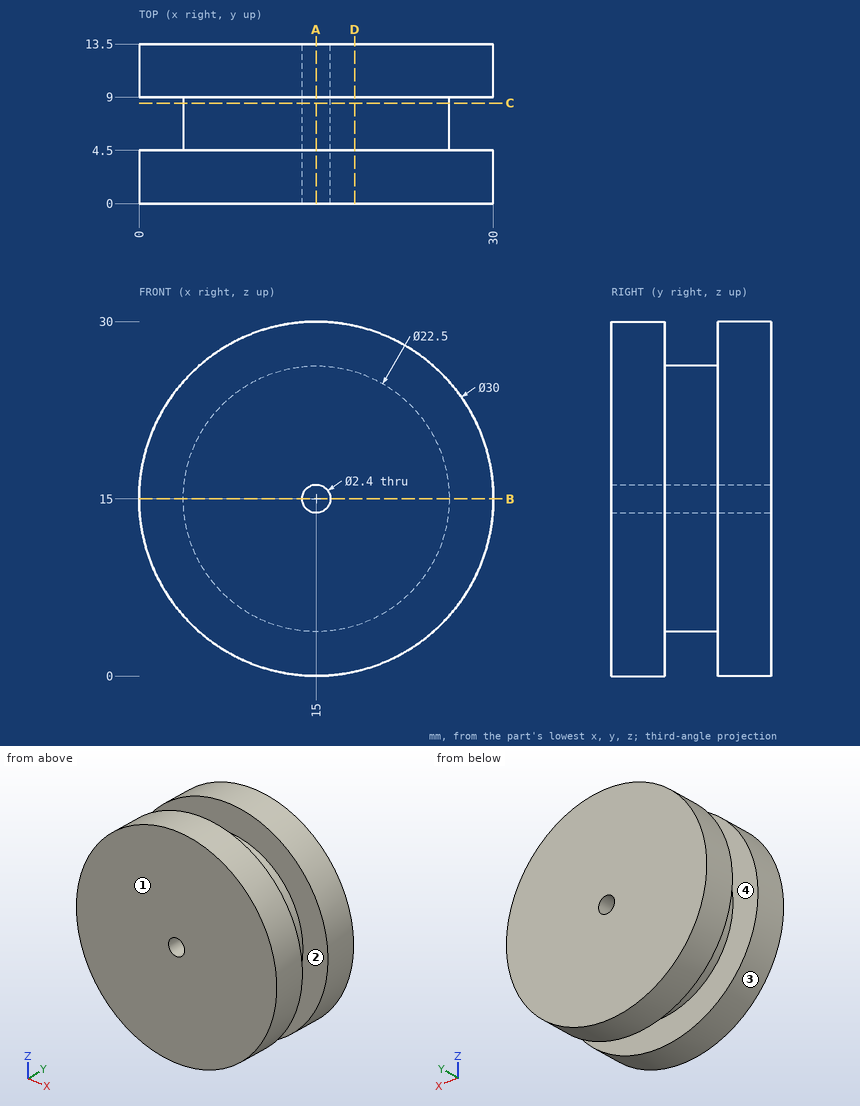
Geometry: see drawing. Coordinates: mm, zero at the bounding-box minimum. Coordinates: 2 decimals unless noted, no trailing zeros. Order: outer loops, then holes, each group sorted by start corner. A loop starts at its lowest first (then second) coordinate and runs counter-clockwise, first axis right, second up. Notation, with made-up numbers: M 82,83 L 98,83 A36 cw 98,121 Z; hole C 8,65.25 d5. An arc over 180 degrees is marked long. Write item = value, one per line. Start each with the question number.
(1) Pull-direction query (Y, two-part tool) for the marked faces 1, 2, 3 and 4; classes: released by +Y, released by -Y, zero draft, split by the parting line, or undercut.
(2) Section C-C on y = 8.5. Output: boundary loops of the cut face in (x, z), and give its area (3 significant figures).
(3) Line query: line 1 along X through (y, z) = (5.25, 15); line 2 along Y through (x, z) = (27.5, 20.5); line 3 along Z through (x, y) = (15, 9.5). Output: solid intervals per line, ascending. Write a range as [from, to].
(4) Section A-A on x = 15. Output: boundary loops of the cut face in (y, z).
(5) Section B-B on z = 15. Output: boundary loops of the cut face in (x, y).
(6) Section D-D on x = 18.25. Output: boundary loops of the cut face in (y, z).
(7) First-contact query: P1, Ø3, axis at x = 15, z = 15, coming from the -Y side; P2, Ø2, axis at x = 18.5, y = 11, coming from the -Z side; P3, Ø2, axis at x = 26, y = 12, coming from the +Z side; P4, Ø3, axis at x = 8, y = 9, coming from the -Z side. Flat tips, straight axial feed; report the tip coordinate or a pass-through.
Result set:
q1.face_1 = released by -Y
q1.face_2 = undercut
q1.face_3 = zero draft
q1.face_4 = undercut
q2.outline = C 15,15 d22.5; hole C 15,15 d2.4
q2.area = 393 mm²
q3.line_1 = [3.75, 13.8], [16.2, 26.25]
q3.line_2 = [0, 4.5], [9, 13.5]
q3.line_3 = [0, 13.8], [16.2, 30]
q4.outline = M 0,0 L 4.5,0 L 4.5,3.75 L 9,3.75 L 9,0 L 13.5,0 L 13.5,13.8 L 0,13.8 Z; M 0,16.2 L 13.5,16.2 L 13.5,30 L 9,30 L 9,26.25 L 4.5,26.25 L 4.5,30 L 0,30 Z
q5.outline = M 0,0 L 13.8,0 L 13.8,13.5 L 0,13.5 L 0,9 L 3.75,9 L 3.75,4.5 L 0,4.5 Z; M 16.2,0 L 30,0 L 30,4.5 L 26.25,4.5 L 26.25,9 L 30,9 L 30,13.5 L 16.2,13.5 Z
q6.outline = M 0,0.36 L 4.5,0.36 L 4.5,4.23 L 9,4.23 L 9,0.36 L 13.5,0.36 L 13.5,29.64 L 9,29.64 L 9,25.77 L 4.5,25.77 L 4.5,29.64 L 0,29.64 Z
q7.P1 = 0
q7.P2 = 0.21
q7.P3 = 26.18
q7.P4 = 1.04
